Here's how the part is built. I have some questions about the finished solid (model axes, mm). Face numbers are marked on the shaded views. A direction names the side the tool comes from. Give positions to 0.01 mm unless a question says otherwise; leave off trailing zeros. Write each loop counter-clockwise with the first axis right and the second up, starting at its lowest first coordinate (ties: lowest second). Pieces come first, ordered by that corner, then holes. Notation, with made-up numbers: (74.25, 48) - (123.25, 48) arc R15 ccw to (123.25, 70) - close; hole circle Ø2 at (70.5, 2). An arc over 180 degrees is marked (long way). Use a Markdown table: item, result.
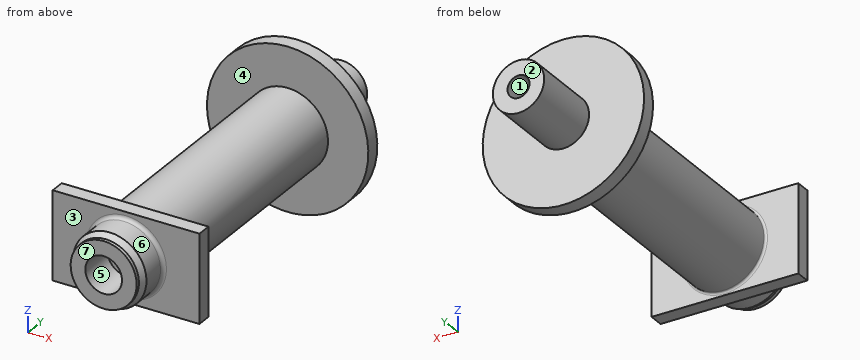
```python
from build123d import *

# Parameters (mm, degrees)
FILLET1_R           = 3
SKETCH3_R           = 25
CUT_EXTRUDE2_DEPTH  = 410
SKETCH4_R           = 15
CUT_EXTRUDE3_DEPTH  = 150
BOSS_EXTRUDE1_DEPTH = 20


with BuildPart() as part:
    # Sketch1 → Revolve1 (revolve)
    with BuildSketch(Plane.XY, mode=Mode.PRIVATE) as revolve1_sk:
        with BuildLine():
            Line((0, 0), (-45, 0))
            Line((-45, 0), (-45, 5))
            Line((-45, 5), (-50, 13.660254038))
            Line((-50, 13.660254038), (-50, 45))
            ThreePointArc((-50, 45), (-51.464466094, 48.535533906), (-55, 50))
            Line((-55, 50), (-60, 50))
            Line((-60, 50), (-60, 70))
            Line((-60, 70), (-55, 70))
            Line((-55, 70), (-55, 410))
            Line((-55, 410), (-110, 410))
            Line((-110, 410), (-110, 430))
            Line((-110, 430), (-35, 430))
            Line((-35, 430), (-35, 530))
            Line((-35, 530), (0, 530))
            Line((0, 530), (0, 0))
        make_face()
    revolve(revolve1_sk.sketch.rotate(Axis((0, 530, 0), (0, -1, 0)), 270), axis=Axis((0, 530, 0), (0, -1, 0)))

    # Fillet1
    fillet1_edges = [part.edges().sort_by_distance(p)[0] for p in [
        (0, 70, -55),
    ]]
    fillet(fillet1_edges, radius=FILLET1_R)

    # Sketch3 → Cut-Extrude2 (cut)
    with BuildSketch(Plane.XZ):
        with Locations(Location((0, 0, 0), (0, 0, 270))):
            Circle(SKETCH3_R)
    extrude(amount=-CUT_EXTRUDE2_DEPTH, mode=Mode.SUBTRACT)

    # Sketch4 → Cut-Extrude3 (cut)
    with BuildSketch(Plane(origin=(0, 530, 0), x_dir=(1, 0, 0), z_dir=(0, 1, 0))):
        with Locations(Location((0, 0, 0), (0, 0, 180))):
            Circle(SKETCH4_R)
    extrude(amount=-CUT_EXTRUDE3_DEPTH, mode=Mode.SUBTRACT)

    # Sketch6 → Boss-Extrude1 (add)
    with BuildSketch(Plane(origin=(0, 50, 0), x_dir=(1, 0, 0), z_dir=(0, 1, 0))):
        Polygon((0, -60), (100, -60), (100, 60), (-100, 60), (-100, -60), align=None)
    extrude(amount=BOSS_EXTRUDE1_DEPTH)


solid = part.part
```
Item 1: Thinking about a two-plate mould opening in Z: for the marked faces 5, 6 and 7, which applies, +Z half, -Z half, draft (parallel to the pull), parting line (faces both ways), or undercut?
Values:
| item | result |
|---|---|
| face 5 | undercut |
| face 6 | parting line |
| face 7 | draft |
Item 2: If we section it at C-C, the plane z = 93: Write out the boundary of the cut face in (x, y).
Values:
| item | result |
|---|---|
| outline | (-58.75, 410) - (58.75, 410) - (58.75, 430) - (-58.75, 430) - close |
Item 3: If we section it at D-D, the plane y = 416.5: Write out the boundary of the cut face in (x, z).
Values:
| item | result |
|---|---|
| outline | circle Ø220 at (0, 0); hole circle Ø30 at (0, 0) |
Item 4: If we section it at B-B, the plane y = 112: Write out the boundary of the cut face in (x, z), plus the area to 3 significant figures.
Values:
| item | result |
|---|---|
| outline | circle Ø110 at (0, 0); hole circle Ø50 at (0, 0) |
| area | 7,540 mm2 |
Item 5: Will these pins go through, and if not, where does the flat tip stop? pin 1 Ø10 at (x, y) = (14.5, 194) entering from -Z; pin 2 Ø6 at (y, z) = (410, 57) entering from +X; pin 3 Ø1 at (x, z) = (54, -71) entering from +Y.
Values:
| item | result |
|---|---|
| pin 1 | stops at z = -54.17 |
| pin 2 | stops at x = 95.83 |
| pin 3 | stops at y = 430 |
Item 6: I need wall thicknesses on line 1 along X through (y, z) = (226, 0); line 2 along Y through (x, z) = (49, -41); line 3 along X through (y, z) = (24, 0). Which ranges of each line are inside material? Lowest first, please. Write a range as [from, to].
Values:
| item | result |
|---|---|
| line 1 | x = [-55, -25], [25, 55] |
| line 2 | y = [50, 70], [410, 430] |
| line 3 | x = [-50, -25], [25, 50] |
Item 7: For the marked faces 1, 2, 3 and 4, which set-ups out of +Z, -Z, +X, -X, +Y, -Y let a thin tool reach every point of the face, with its end or its side?
Values:
| item | result |
|---|---|
| face 1 | +Y |
| face 2 | +Z, -Z, +X, -X, +Y |
| face 3 | -Y |
| face 4 | none |
Item 8: If we section it at A-A, the plane x = 71: Write out the boundary of the cut face in (y, z).
Values:
| item | result |
|---|---|
| outline | (50, -60) - (70, -60) - (70, 60) - (50, 60) - close; (410, -84.02) - (430, -84.02) - (430, 84.02) - (410, 84.02) - close |
